```python
from build123d import *

# Parameters (mm, degrees)
SKETCH_1_R               = 10
SKETCH_1_R_2             = 8.75
EXTRUDE_1_DEPTH          = 120
SKETCH_2_R               = 3.1
CUT_EXTRUDE_1_DEPTH      = 11
CUT_EXTRUDE_1_DEPTH_BACK = 11


with BuildPart() as part:
    # 草图1 → 凸台-拉伸1 (new body)
    with BuildSketch(Plane(origin=(0, 0, 0), x_dir=(0, 0, -1), z_dir=(1, 0, 0))):
        Circle(SKETCH_1_R)
        Circle(SKETCH_1_R_2, mode=Mode.SUBTRACT)
    extrude(amount=EXTRUDE_1_DEPTH)

    # 草图2 → 切除-拉伸1 (cut, two sides)
    with BuildSketch(Plane(origin=(0, 0, 0), x_dir=(1, 0, 0), z_dir=(0, 1, 0))) as cut_extrude_1_sk:
        with Locations((20, 0)):
            Circle(SKETCH_2_R)
        with Locations((100, 0)):
            Circle(SKETCH_2_R)
    extrude(amount=CUT_EXTRUDE_1_DEPTH, mode=Mode.SUBTRACT)
    extrude(cut_extrude_1_sk.sketch, amount=-CUT_EXTRUDE_1_DEPTH_BACK, mode=Mode.SUBTRACT)


solid = part.part
```
Source: CAD feature listing. Evaluate the final solid. Frame: model axes, mm. Coordinates: 2 decimals unless noted, no trailing zeros. Write each loop counter-clockwise with the first axis right and the second up, starting at its lowest first coordinate (ties: lowest second). Pieces come first, ordered by that corner, then holes. Notation, with made-up numbers: M -21,-12 L 26,-12 A15 ccw 26,8 Z; hole C 6,51.5 d4. An arc over 180 degrees is marked long. Answer as a JSON object with one key per item and string values.
1. Contact query for flat-ended pins moving along their axis: P1, Ø10, axis at x = 82.5, z = 7, coming from the +Y side; P2, Ø10, axis at x = 90, y = 5.5, coming from the -Z side; P3, Ø5, axis at x = 64, y = 6.5, coming from the -Z side. Output: stop coordinate, or through.
Evaluation:
{"P1": "y = 9.8", "P2": "z = -9.99", "P3": "z = -9.17"}
2. Cut plane B-B on z = 0. Output: boundary loops of the cut face in (x, y), plus the area to 3 significant figures.
Evaluation:
{"outline": "M 0,-10 L 16.9,-10 L 16.9,-8.75 L 0,-8.75 Z; M 0,8.75 L 16.9,8.75 L 16.9,10 L 0,10 Z; M 23.1,-10 L 96.9,-10 L 96.9,-8.75 L 23.1,-8.75 Z; M 23.1,8.75 L 96.9,8.75 L 96.9,10 L 23.1,10 Z; M 103.1,-10 L 120,-10 L 120,-8.75 L 103.1,-8.75 Z; M 103.1,8.75 L 120,8.75 L 120,10 L 103.1,10 Z", "area": "269 mm^2"}
3. Cut plane C-C on x = 20. Output: boundary loops of the cut face in (y, z), plus the area to 3 significant figures.
Evaluation:
{"outline": "M -9.51,-3.1 A10 ccw 9.51,-3.1 L 8.18,-3.1 A8.75 cw -8.18,-3.1 Z; M -9.51,3.1 L -8.18,3.1 A8.75 cw 8.18,3.1 L 9.51,3.1 A10 ccw Z", "area": "57.8 mm^2"}
4. Draft query along Y for faces 1 (the flat face through (120, -9, 0)), 2 (the cylindrical face through (59.16, -3.83, -9.237)), 3 (the cylindrical face through (59.16, -3.351, -8.083)). Return one class per face: released by +Y, released by -Y, zero draft, split by the parting line, or undercut.
Evaluation:
{"face 1": "zero draft", "face 2": "split by the parting line", "face 3": "undercut"}
5. Cut plane A-A on y = 0. Output: boundary loops of the cut face in (x, z).
Evaluation:
{"outline": "M 0,-10 L 120,-10 L 120,-8.75 L 0,-8.75 Z; M 0,8.75 L 120,8.75 L 120,10 L 0,10 Z"}
6. Ray query, L1, parallel to X at y = -9.55, z = 0; L2, parallel to Z at x = 100, y = -0.5; L3, parallel to Y at x = 19, z = 5.5. Return the intervals inside material, ascending.
Evaluation:
{"L1": "0 to 16.9, 23.1 to 96.9, 103.1 to 120", "L2": "-9.99 to -8.74, 8.74 to 9.99", "L3": "-8.35 to -6.81, 6.81 to 8.35"}
